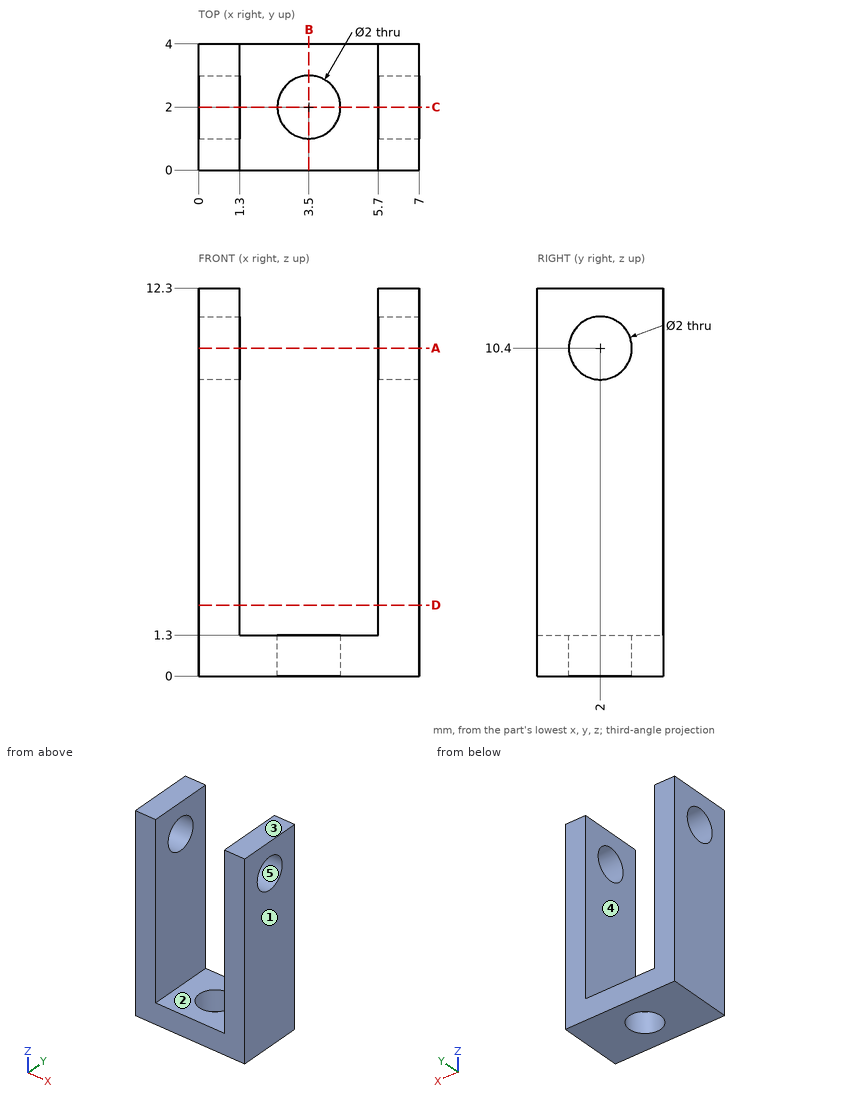
Check sheet for the drawn part. Datum: minimum x, y, z corner. Units: mm. A direction names the side the tool comes from. Round coordinates to 2 decimals unless told otherwise and drop trailing zeros. Order: outer loops, then holes, each group sorted by start corner. A loop starts at its lowest first (then second) coordinate and runs counter-clockwise, first axis right, second up. Notation, with made-up numbers: M 11,73.25 L 63,73.25 A25 cw 63,93.25 Z; hole C 17,45 d4. An arc over 180 degrees is marked long. Answer in a Markdown table with one row per item.
(1) Gauge pin test, flat ends, axial feed: pin 1 (1.2 mm diameter, centred on y = 2.5, z = 8.5, fed in from -X); pin 2 (1.6 mm diameter, centred on y = 2, z = 10.4, fed in from -X); pin 3 (1.2 mm diameter, centred on x = 3, y = 1, fed in from +Z). Record the tip position at first contact, or that the pin passes through.
Findings:
| item | result |
|---|---|
| pin 1 | stops at x = 0 |
| pin 2 | passes through |
| pin 3 | stops at z = 1.3 |
(2) Draft check along X on the marked faces 1, 2 and 3. Enter one of: +X half, -X half, draft (parallel to the pull), parting line (faces both ways), or undercut.
Findings:
| item | result |
|---|---|
| face 1 | +X half |
| face 2 | undercut |
| face 3 | draft |
(3) Set-up check for the marked faces 4 and 5: record each of +Z, -Z, +X, -X, +Y, -Y from which the full face is reachable in a straight line by a thin tool's end or side.
Findings:
| item | result |
|---|---|
| face 4 | +Z, +Y, -Y |
| face 5 | +X, -X |
(4) Section check A-A on z = 10.4. Record the boundary of the cut face in (x, y), plus the area to 3 significant figures.
Findings:
| item | result |
|---|---|
| outline | M 0,0 L 1.3,0 L 1.3,1 L 0,1 Z; M 0,3 L 1.3,3 L 1.3,4 L 0,4 Z; M 5.7,0 L 7,0 L 7,1 L 5.7,1 Z; M 5.7,3 L 7,3 L 7,4 L 5.7,4 Z |
| area | 5.20 mm^2 |
(5) Section check D-D on z = 2.25. Record the boundary of the cut face in (x, y).
Findings:
| item | result |
|---|---|
| outline | M 0,0 L 1.3,0 L 1.3,4 L 0,4 Z; M 5.7,0 L 7,0 L 7,4 L 5.7,4 Z |
(6) Section check B-B on x = 3.5. Record the boundary of the cut face in (y, z).
Findings:
| item | result |
|---|---|
| outline | M 0,0 L 1,0 L 1,1.3 L 0,1.3 Z; M 3,0 L 4,0 L 4,1.3 L 3,1.3 Z |
(7) Section check C-C on y = 2. Record the boundary of the cut face in (x, z).
Findings:
| item | result |
|---|---|
| outline | M 0,0 L 2.5,0 L 2.5,1.3 L 1.3,1.3 L 1.3,9.4 L 0,9.4 Z; M 0,11.4 L 1.3,11.4 L 1.3,12.3 L 0,12.3 Z; M 4.5,0 L 7,0 L 7,9.4 L 5.7,9.4 L 5.7,1.3 L 4.5,1.3 Z; M 5.7,11.4 L 7,11.4 L 7,12.3 L 5.7,12.3 Z |
(8) Material ranges on line 1 along Y through (x, z) = (6.75, 10.4); line 2 along X through (y, z) = (2.75, 2.25); line 3 along Z through (x, y) = (4.5, 3.6), recorded low to high. Write a range as from..to.
Findings:
| item | result |
|---|---|
| line 1 | y = 0..1, 3..4 |
| line 2 | x = 0..1.3, 5.7..7 |
| line 3 | z = 0..1.3 |
